The figure shows three views and two pictorial views of one solid part (mm, origin at its lowest corner). Answer the questions. Coordinates: 2 decimals unless noted, no trailing zeros. Loops run counter-clockwise (first coordinate to the right, second up) from the corner with the lowest first, then second, coordinate; pieces in that order, holes last. Notation, with made-up numbers: (-23.75, 88) - (7.25, 88) arc R22 cw to (7.25, 103) - close; hole circle Ø9 at (59, 62.25). An arc over 180 degrees is marked (long way). Return JSON: item names as keys, results as strings. Group by question number.
1. The mould has two halves that part along Z. Classify the marked faces 1, 2 and 3: pulls with the +Z half, pulls with the -Z half, needs draft (parallel to the pull), parting line crosses it, or undercut.
2. Section D-D (z = 7) is taken. Write down the section's boundary in (x, y).
3. Section C-C (x = 21.5) is taken. Write down the section's boundary in (y, z), and give its area (3 significant figures).
4. Find the intervals of material crossed by line 1 along Z through (x, y) = (21.5, 1.65); line 2 along X through (y, z) = (3.7, 9.75); line 3 along X through (y, z) = (1.2, 6), in increasing order.
5. Section B-B (z = 8.5) is taken. Write down the section's boundary in (x, y), and give its area (3 significant figures).
6. Section A-A (y = 4.45) is taken. Write down the section's boundary in (x, z).
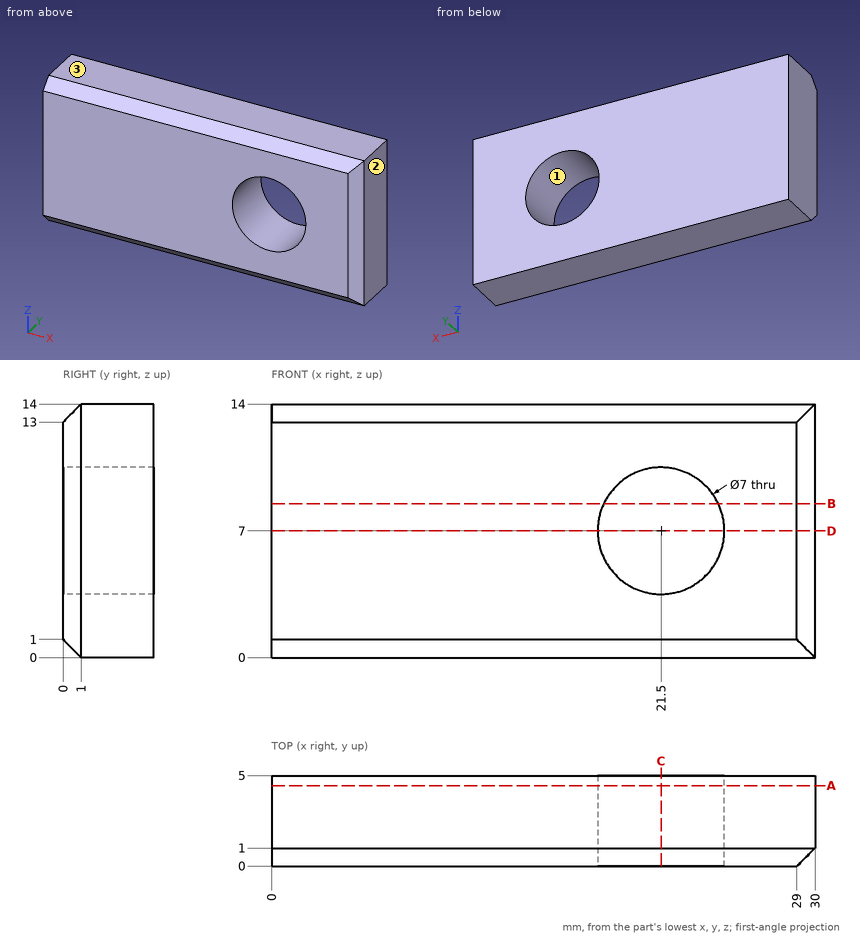
The answers:
{
 "1": {"face 1": "undercut", "face 2": "needs draft", "face 3": "pulls with the +Z half"},
 "2": {"outline": "(0, 0) - (18, 0) - (18, 5) - (0, 5) - close; (25, 0) - (29, 0) - (30, 1) - (30, 5) - (25, 5) - close"},
 "3": {"outline": "(0, 1) - (1, 0) - (5, 0) - (5, 3.5) - (0, 3.5) - close; (0, 10.5) - (5, 10.5) - (5, 14) - (1, 14) - (0, 13) - close", "area": "34.0 mm2"},
 "4": {"line 1": "z = 0 to 3.5, 10.5 to 14", "line 2": "x = 0 to 19.33, 23.67 to 30", "line 3": "x = 0 to 18.15, 24.85 to 30"},
 "5": {"outline": "(0, 0) - (18.34, 0) - (18.34, 5) - (0, 5) - close; (24.66, 0) - (29, 0) - (30, 1) - (30, 5) - (24.66, 5) - close", "area": "118 mm2"},
 "6": {"outline": "(0, 0) - (30, 0) - (30, 14) - (0, 14) - close; hole circle Ø7 at (21.5, 7)"}
}
